For this review, take the finished solid that the model builds, in its own axes (mm). Face numbers are marked on the shaded views. A direction names the side the tool comes from. Coordinates: 2 decimals unless noted, no trailing zeros. Order: outer loops, then holes, each group sorted by start corner. A loop starts at its lowest first (then second) coordinate and runs counter-clockwise, first axis right, second up. Notation, with made-up numbers: M 23.25,65 L 29.25,65 A19 ccw 29.25,84 Z; hole C -2.5,-16.5 d9. An arc over 180 degrees is marked long. Use CSV: the item, a comma, the result in double quotes.
```python
from build123d import *

# Parameters (mm, degrees)
SKETCH1_R           = 11
SKETCH1_R_2         = 5
SKETCH1_R_3         = 2.5
BOSS_EXTRUDE1_DEPTH = 2
SKETCH1_3_R         = 5
SKETCH1_3_R_2       = 2.5
BOSS_EXTRUDE2_DEPTH = 12
SKETCH2_R           = 1.425
CUT_EXTRUDE1_DEPTH  = 19.493242009
CIRPATTERN1_COUNT   = 4


with BuildPart() as part:
    # Sketch1 → Boss-Extrude1 (new body)
    # profile 1 of 2: a face of its own
    with BuildSketch(Plane(origin=(0, 0, 0), x_dir=(1, 0, 0), z_dir=(0, 1, 0))):
        with Locations(Location((0, 0, 0), (0, 0, 270))):
            Circle(SKETCH1_R)
        Circle(SKETCH1_R_2, mode=Mode.SUBTRACT)
    # profile 2 of 2: a face of its own
    with BuildSketch(Plane(origin=(0, 0, 0), x_dir=(1, 0, 0), z_dir=(0, 1, 0))):
        Circle(SKETCH1_R_2)
        with Locations(Location((0, 0, 0), (0, 0, 270))):
            Circle(SKETCH1_R_3, mode=Mode.SUBTRACT)
    extrude(amount=BOSS_EXTRUDE1_DEPTH)

    # Sketch1_3 → Boss-Extrude2 (add)
    with BuildSketch(Plane(origin=(0, 0, 0), x_dir=(1, 0, 0), z_dir=(0, 1, 0))):
        with Locations(Location((0, 0, 0), (0, 0, 270))):
            Circle(SKETCH1_3_R)
        with Locations(Location((0, 0, 0), (0, 0, 270))):
            Circle(SKETCH1_3_R_2, mode=Mode.SUBTRACT)
    extrude(amount=BOSS_EXTRUDE2_DEPTH)

    # Sketch2 → Cut-Extrude1 (cut, symmetric)
    with BuildSketch(Plane(origin=(0, 2, 0), x_dir=(1, 0, 0), z_dir=(0, 1, 0))):
        with Locations(Location((0, 8, 0), (0, 0, 270))):
            Circle(SKETCH2_R)
    cut_extrude1 = extrude(amount=CUT_EXTRUDE1_DEPTH, both=True, mode=Mode.SUBTRACT)

    # CirPattern1: Cut-Extrude1 ×4 about axis
    cirpattern1_axis = Axis((0, 0, 0), (0, 1, 0))
    for i in range(1, CIRPATTERN1_COUNT):
        add(cut_extrude1.rotate(cirpattern1_axis, i * 360 / CIRPATTERN1_COUNT), mode=Mode.SUBTRACT)


solid = part.part
```
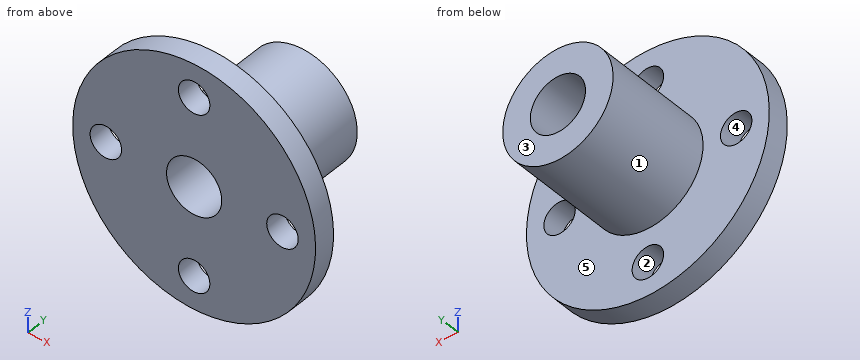
Item 1: Add section D-D on x = -7.75. State the section outline as (y, z) points.
Solutions:
outline,"M 0,-7.81 L 2,-7.81 L 2,-1.4 L 0,-1.4 Z; M 0,1.4 L 2,1.4 L 2,7.81 L 0,7.81 Z"
Item 2: To check wall thickness, follow line 1 along Y through (x, z) = (2.25, 4.5); line 2 along Z through (x, y) = (-1, 0.5); line 3 along Z through (x, y) = (-2, 2.75). State the ranges of each line that lie inside material, in increasing order. Write a range as [from, to].
Solutions:
line 1,"[0, 2]"
line 2,"[-10.95, -9.02], [-6.98, -2.29], [2.29, 6.98], [9.02, 10.95]"
line 3,"[-4.58, -1.5], [1.5, 4.58]"
Item 3: Draft analysis for pull direction X (two halves, no side actions). For the marked faces 1, 2 and 3, state which applies: released by +X, released by -X, zero draft, split by the parting line, or undercut.
Solutions:
face 1,"split by the parting line"
face 2,"undercut"
face 3,"zero draft"
Item 4: Add section B-B on z = 8. State the section outline as (x, y) points (3 decimals).
Solutions:
outline,"M -7.55,0 L -1.425,0 L -1.425,2 L -7.55,2 Z; M 1.425,0 L 7.55,0 L 7.55,2 L 1.425,2 Z"
Item 5: Add section C-C on z = 0. State the section outline as (x, y) points (3 decimals).
Solutions:
outline,"M -11,0 L -9.425,0 L -9.425,2 L -11,2 Z; M -6.575,0 L -2.5,0 L -2.5,12 L -5,12 L -5,2 L -6.575,2 Z; M 2.5,0 L 6.575,0 L 6.575,2 L 5,2 L 5,12 L 2.5,12 Z; M 9.425,0 L 11,0 L 11,2 L 9.425,2 Z"
Item 6: Add section A-A on x = 0. State the section outline as (y, z) points (3 decimals).
Solutions:
outline,"M 0,-11 L 2,-11 L 2,-9.425 L 0,-9.425 Z; M 0,-6.575 L 2,-6.575 L 2,-5 L 12,-5 L 12,-2.5 L 0,-2.5 Z; M 0,2.5 L 12,2.5 L 12,5 L 2,5 L 2,6.575 L 0,6.575 Z; M 0,9.425 L 2,9.425 L 2,11 L 0,11 Z"
Item 7: Clearance check with flat-ended pins moving along their axes: pin 1 Ø3 at (y, z) = (2.5, 1.5) entering from -X; pin 2 Ø1.5 at (y, z) = (6, 1) entering from +X; pin 3 Ø6 at (x, y) = (-6, 3) entering from -Z; pin 4 Ø2.5 at (x, z) = (0, 8) entering from -Y. State where each tip first meets the part, or that it passes through.
Solutions:
pin 1,"x = -11"
pin 2,"x = 4.99"
pin 3,"z = -10.53"
pin 4,"through"
Item 8: For the marked faces 4 and 5, list the 3-axis set-ups (+Z, -Z, +X, -X, +Y, -Y) from which the entire face can be reached by the end or side of a thin tool; tool diameter is ignored.
Solutions:
face 4,"+Y, -Y"
face 5,"+Y"
